Input: part model. Units: mm. Frame: model coordinates. Face numbers are marked on the shaded views. Give positions to 0.01 mm unless a question says otherwise; leave off trailing zeros. Loops run counter-clockwise (first coordinate to the right, second up) from the corner with the lowest first, then second, coordinate; pieces in that order, holes last. Notation, with made-up numbers: M -5,-5 L 29,-5 A12 ccw 29,5 Z; hole C 55,-24 d3. An arc over 180 degrees is marked long. One line per item, written item: value. Start each with the question number.
(1) Section A-A on z = 73. Output: boundary loops of the cut face in (x, y).
(2) Section B-B on x = 139.5. Output: boundary loops of the cut face in (y, z), plus the area to 3 significant figures.
(3) Pull-direction query (X, two-part tool) for the marked faces 1 and 2; classes: released by +X, released by -X, zero draft, split by the parting line, or undercut.
(4) Ray query, line 1 along Z through (x, y) = (151.7, 1.3); line 2 along X through (y, z) = (-5.25, -143); line 3 along X through (y, z) = (0.6, -161). Return the intervals inside material, ascending. Write a range as from..to.
(5) Pin query (flat end, axial travel): P1, Ø6, axis at x = 0, z = 161, coming from the +Y side; P2, Ø2, axis at x = 194.5, z = -133, coming from the -Y side; P3, Ø6.5, axis at x = 186.46, z = 124.5, coming from the -Y side; P4, Ø1.9, axis at x = -193.5, y = -11, coming from the -Z side. Return the tip coordinate at first contact, or that it passes through.
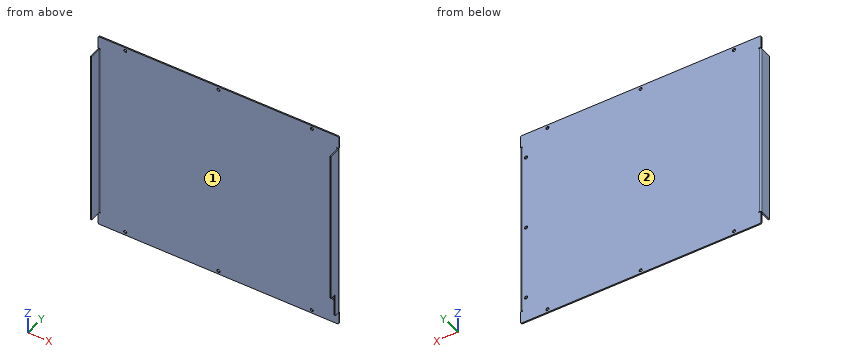
```python
from build123d import *

# Parameters (mm, degrees)
SKETCH1_W                       = 391.4
SKETCH1_H                       = 333
BASE_FLANGE1_DEPTH              = 2
EDGE_FLANGE1_STRIP_W            = 9.4732
EDGE_FLANGE1_STRIP_H            = 2
EDGE_FLANGE1_STRIP_CUT_DEPTH    = 290
EDGE_FLANGE1_RELIEF_W           = 10.4732
EDGE_FLANGE1_RELIEF_H           = 1
EDGE_FLANGE1_RELIEF_CUT_DEPTH   = 2
EDGE_FLANGE1_STRIP_2_W          = 9.4732
EDGE_FLANGE1_STRIP_2_H          = 2
EDGE_FLANGE1_STRIP_CUT_2_DEPTH  = 290
EDGE_FLANGE1_RELIEF_2_W         = 10.4732
EDGE_FLANGE1_RELIEF_2_H         = 1
EDGE_FLANGE1_RELIEF_CUT_2_DEPTH = 2
EDGE_FLANGE1_DEPTH              = 290
EDGE_FLANGE1_BEND_DEPTH         = 290
FILLET1_R                       = 2
CUT_EXTRUDE1_DEPTH              = 10
FILLET2_R                       = 1
CUT_EXTRUDE2_DEPTH              = 258.84295608
CUT_EXTRUDE2_DEPTH_BACK         = 258.84295608
SKETCH9_R                       = 2.5


# Sheet-metal steps are written as plain solids
with BuildPart() as part:
    # Sketch1 → Base-Flange1 (new body)
    with BuildSketch(Plane(origin=(0, 0, 0), x_dir=(1, 0, 0), z_dir=(0, 1, 0))):
        Rectangle(SKETCH1_W, SKETCH1_H)
    extrude(amount=BASE_FLANGE1_DEPTH)

    # Edge-Flange1 strip (across the edge) → Edge-Flange1 strip cut (cut)
    with BuildSketch(Plane(origin=(-195.7, 0, 145), x_dir=(1, 0, 0), z_dir=(0, 0, -1))):
        with Locations((-2, -1)):
            Rectangle(EDGE_FLANGE1_STRIP_W, EDGE_FLANGE1_STRIP_H)
    extrude(amount=EDGE_FLANGE1_STRIP_CUT_DEPTH, mode=Mode.SUBTRACT)

    # Edge-Flange1 relief (on the sheet) → Edge-Flange1 relief cut (cut)
    with BuildSketch(Plane(origin=(-192.9634, 0, 145), x_dir=(1, 0, 0), z_dir=(0, -1, 0))):
        with Locations((-4.2366, 0.5)):
            Rectangle(EDGE_FLANGE1_RELIEF_W, EDGE_FLANGE1_RELIEF_H)
        with Locations((-4.2366, -290.5)):
            Rectangle(EDGE_FLANGE1_RELIEF_W, EDGE_FLANGE1_RELIEF_H)
    extrude(amount=-EDGE_FLANGE1_RELIEF_CUT_DEPTH, mode=Mode.SUBTRACT)

    # Edge-Flange1 strip 2 (across the edge) → Edge-Flange1 strip cut 2 (cut)
    with BuildSketch(Plane(origin=(195.7, 0, -145), x_dir=(-1, 0, 0), z_dir=(0, 0, 1))):
        with Locations((-2, -1)):
            Rectangle(EDGE_FLANGE1_STRIP_2_W, EDGE_FLANGE1_STRIP_2_H)
    extrude(amount=EDGE_FLANGE1_STRIP_CUT_2_DEPTH, mode=Mode.SUBTRACT)

    # Edge-Flange1 relief 2 (on the sheet) → Edge-Flange1 relief cut 2 (cut)
    with BuildSketch(Plane(origin=(192.9634, 0, -145), x_dir=(-1, 0, 0), z_dir=(0, -1, 0))):
        with Locations((-4.2366, 0.5)):
            Rectangle(EDGE_FLANGE1_RELIEF_2_W, EDGE_FLANGE1_RELIEF_2_H)
        with Locations((-4.2366, -290.5)):
            Rectangle(EDGE_FLANGE1_RELIEF_2_W, EDGE_FLANGE1_RELIEF_2_H)
    extrude(amount=-EDGE_FLANGE1_RELIEF_CUT_2_DEPTH, mode=Mode.SUBTRACT)

    # Edge-Flange1 section (across the edge) → Edge-Flange1 (add)
    with BuildSketch(Plane(origin=(-195.7, 0, 145), x_dir=(1, 0, 0), z_dir=(0, 0, -1))):
        with BuildLine():
            Line((0, 0.7366), (0, 19.5))
            Line((0, 19.5), (2, 19.5))
            Line((2, 19.5), (2, 0.7366))
            ThreePointArc((2, 0.7366), (2.215745145, 0.215745145), (2.7366, 0))
            Line((2.7366, 0), (2.7366, -2))
            ThreePointArc((2.7366, -2), (0.801531583, -1.198468417), (0, 0.7366))
        make_face()
    extrude(amount=EDGE_FLANGE1_DEPTH)

    # Edge-Flange1 section 2 (across the edge) → Edge-Flange1 bend (add)
    with BuildSketch(Plane(origin=(195.7, 0, -145), x_dir=(-1, 0, 0), z_dir=(0, 0, 1))):
        with BuildLine():
            Line((0, 0.7366), (0, 19.5))
            Line((0, 19.5), (2, 19.5))
            Line((2, 19.5), (2, 0.7366))
            ThreePointArc((2, 0.7366), (2.215745145, 0.215745145), (2.7366, 0))
            Line((2.7366, 0), (2.7366, -2))
            ThreePointArc((2.7366, -2), (0.801531583, -1.198468417), (0, 0.7366))
        make_face()
    extrude(amount=EDGE_FLANGE1_BEND_DEPTH)

    # Fillet1
    fillet1_edges = [part.edges().sort_by_distance(p)[0] for p in [
        (195.7, 1, 166.5),
        (-195.7, 1, 166.5),
        (-195.7, 1, -166.5),
        (195.7, 1, -166.5),
    ]]
    fillet(fillet1_edges, radius=FILLET1_R)

    # Sketch8 → Cut-Extrude1 (cut)
    with BuildSketch(Plane(origin=(195.7, 0, 0), x_dir=(0, 0, -1), z_dir=(1, 0, 0))):
        with BuildLine():
            Line((107.5, -19.5), (147.855530229, -19.5))
            Line((147.855530229, -19.5), (147.855530229, -9))
            Line((147.855530229, -9), (108.5, -9))
            ThreePointArc((108.5, -9), (107.792893219, -9.292893219), (107.5, -10))
            Line((107.5, -10), (107.5, -19.5))
        make_face()
    extrude(amount=-CUT_EXTRUDE1_DEPTH, mode=Mode.SUBTRACT)

    # Fillet2
    fillet2_edges = [part.edges().sort_by_distance(p)[0] for p in [
        (194.7, -19.5, -107.5),
        (194.7, -9, -145),
    ]]
    fillet(fillet2_edges, radius=FILLET2_R)

    # Sketch9 → Cut-Extrude2 (cut, two sides: drawn at the far end of the back side and taken through both)
    with BuildSketch(Plane(origin=(0, 2, 0), x_dir=(1, 0, 0), z_dir=(0, 1, 0)).offset(-CUT_EXTRUDE2_DEPTH_BACK)):
        with Locations(Location((-151.7, -161, 0), (0, 0, 270))):
            Circle(SKETCH9_R)
        with Locations(Location((0, -161, 0), (0, 0, 270))):
            Circle(SKETCH9_R)
        with Locations(Location((151.7, -161, 0), (0, 0, 270))):
            Circle(SKETCH9_R)
        with Locations(Location((186.4634, -124.5, 0), (0, 0, 270))):
            Circle(SKETCH9_R)
        with Locations(Location((186.4634, 0, 0), (0, 0, 270))):
            Circle(SKETCH9_R)
        with Locations(Location((186.4634, 124.5, 0), (0, 0, 270))):
            Circle(SKETCH9_R)
        with Locations(Location((151.7, 161, 0), (0, 0, 270))):
            Circle(SKETCH9_R)
        with Locations(Location((0, 161, 0), (0, 0, 270))):
            Circle(SKETCH9_R)
        with Locations(Location((-151.7, 161, 0), (0, 0, 270))):
            Circle(SKETCH9_R)
    extrude(amount=CUT_EXTRUDE2_DEPTH + CUT_EXTRUDE2_DEPTH_BACK, mode=Mode.SUBTRACT)


solid = part.part
```
Output values:
1. outline: M -195.7,-19.5 L -193.7,-19.5 L -193.7,-0.74 A0.74 cw -192.96,0 L 192.96,0 A0.74 cw 193.7,-0.74 L 193.7,-19.5 L 195.7,-19.5 L 195.7,-0.74 A2.74 ccw 192.96,2 L -192.96,2 A2.74 ccw -195.7,-0.74 Z
2. outline: M 0,-166.5 L 2,-166.5 L 2,166.5 L 0,166.5 Z
2. area: 666 mm²
3. face 1: undercut
3. face 2: zero draft
4. line 1: z = -166.5..-163.5, -158.5..158.5, 163.5..166.5
4. line 2: x = -195.7..-193.7, 193.7..195.7
4. line 3: x = -195.7..-154.2, -149.2..-2.5, 2.5..149.2, 154.2..195.7
5. P1: stops at y = 2
5. P2: stops at y = -9
5. P3: stops at y = 0
5. P4: stops at z = -145
